Read the model definition and answer for the solid it produces. Units are mm, in the model's axes. A direction names the side the tool comes from. Coordinates: 2 decimals unless noted, no trailing zeros. Loops run counter-clockwise (first coordinate to the right, second up) from the corner with the lowest first, then second, coordinate; pieces in that order, holes last. Notation, with made-up numbers: (73.25, 12.5) - (101.25, 12.5) arc R12 ccw to (101.25, 29.5) - close; hole circle Ø10 at (3, -8). An arc over 180 degrees is marked (long way). Use one line per item in the form item = value. Start each with the question number.
1) A cutting plane is placed at D-D (x = 15.5). Give the vertices of the cut face in (y, z) (3 decimals).
2) Each of these flat-tipped pins is pushed along its axis until it touches: P1, Ø4, axis at y = 0, z = 0, coming from the +X side; P2, Ø8, axis at x = 11, y = -18, coming from the +Z side; P3, Ø8, axis at y = -10, z = -4, coming from the +X side (3 decimals); P4, Ø4, axis at x = -1, y = 0.5, coming from the -Z side. Where does it stop, or does it pass through?
3) Which of the six approach directions +Z, -Z, +X, -X, +Y, -Y give full straight-line access (tool end or side, diameter ignored) to faces 1 (the face through (-1, 0, -5.08)), 2 (the face through (14, 0, 5.08)), 3 (the face through (-6.35, -3, 2)), 4 (the face through (3.81, -3, 2))?
4) The mould has two halves that part along X. Classify faces 5 (the face through (19.05, -3, -2)), 6 (the face through (13.9, 4.1, 4.2)), 7 (the face through (6, -5.08, 0)): released by +X, released by -X, zero draft, split by the parting line, or undercut.
5) A cutting plane is placed at C-C (x = 10). Give the vertices of the cut face in (y, z) (3 decimals).
6) A cutting plane is placed at A-A (x = 6.35). Give the vertices of the cut face in (y, z) (3 decimals), and give its area (3 significant figures).
7) Consider line 1 (Y direction, x = 16, z = 0) (3 decimals); line 2 (X direction, y = -4, z = -5); line 3 (Z direction, x = 16, y = 0) (3 decimals). Determine where each line is inside the solid, lowest interval first.
Autodesk Inventor part; units mm, degrees
ref_plane "YZ Plane" through (0, 0, 0) normal (1, 0, 0) x (0, 1, 0)
ref_plane "XZ Plane" through (0, 0, 0) normal (0, 1, 0) x (-1, 0, 0)
ref_plane "XY Plane" through (0, 0, 0) normal (0, 0, 1) x (1, 0, 0)
sketch "Sketch1" plane through (0, 0, 0) normal (1, 0, 0) x (0, 1, 0)
  circle A0 centre (0, 0) radius 3.175
  line L0 (-5.08, 5.08) -> (5.08, 5.08)
  line L1 (5.08, 5.08) -> (5.08, -5.08)
  line L2 (5.08, -5.08) -> (-5.08, -5.08)
  line L3 (-5.08, -5.08) -> (-5.08, 5.08)
  line L4 (-5.08, 5.08) -> (5.08, -5.08) construction
  line L5 (5.08, 5.08) -> (-5.08, -5.08) construction
  dimension "d0" = 6.35
  dimension "d1" = 10.16
  dimension "d2" = 10.16
extrude "Extrusion1" add sketch "Sketch1" along normal blind 12.7
sketch "Sketch2" plane through (0, -5.08, -5.08) normal (0, -1, 0) x (1, 0, 0)
  line L0 (-19.05, 30.48) -> (31.75, 30.48)
  line L1 (31.75, 30.48) -> (31.75, -20.32)
  line L2 (31.75, -20.32) -> (-19.05, -20.32)
  line L3 (-19.05, -20.32) -> (-19.05, 30.48)
  line L4 (-19.05, 30.48) -> (31.75, -20.32) construction
  line L5 (31.75, 30.48) -> (-19.05, -20.32) construction
  circle A0 centre (6.35, 5.08) radius 15.875
  point P0 (0, 5.08)
  dimension "d7" = 50.8
  dimension "d8" = 50.8
  dimension "d9" = 31.75
extrude "Extrusion2" add sketch "Sketch2" along normal blind 6.35 contours A0
sketch "Sketch3" plane through (0, 5.08, 5.08) normal (0, 1, 0) x (1, 0, 0)
  line L0 (8.89, 17.78) -> (3.81, 17.78)
  line L1 (3.81, 17.78) -> (3.81, -7.62)
  line L2 (3.81, -7.62) -> (8.89, -7.62)
  line L3 (8.89, -7.62) -> (8.89, 17.78)
  line L4 (8.89, 17.78) -> (3.81, -7.62) construction
  line L5 (3.81, 17.78) -> (8.89, -7.62) construction
  line L6 (12.7, 10.16) -> (12.7, 0)
  point P0 (0, 5.08)
  point P1 (6.35, 5.08)
  dimension "d12" = 5.08
  dimension "d13" = 25.4
  dimension "d42" = 6.35
extrude "Extrusion3" cut sketch "Sketch3" against normal up to surface (10.16 mm away)
sketch "Sketch5" plane through (12.7, 0, 0) normal (1, 0, 0) x (0, 0, -1)
  line L0 (5.08, -5.08) -> (5.08, 5.08)
  line L1 (5.08, 5.08) -> (-5.08, 5.08)
  line L2 (-5.08, 5.08) -> (-5.08, -5.08)
  line L3 (-5.08, -5.08) -> (5.08, -5.08)
  circle A0 centre (0, 0) radius 3.175
extrude "Extrusion4" add sketch "Sketch5" along normal blind 6.35
sketch "Sketch6" plane through (0, 0, 0) normal (-1, 0, 0) x (0, 0, 1)
  line L0 (-5.08, -5.08) -> (-5.08, 5.08)
  line L1 (5.08, -5.08) -> (-5.08, -5.08)
  line L2 (5.08, 5.08) -> (5.08, -5.08)
  line L3 (-5.08, 5.08) -> (5.08, 5.08)
  circle A0 centre (0, 0) radius 3.175
extrude "Extrusion5" add sketch "Sketch6" along normal blind 6.35
fillet "Fillet3" radius 3.175 4 edges at (-1.27, 5.08, -5.08) (13.97, 5.08, -5.08) (-1.27, 5.08, 5.08) (13.97, 5.08, 5.08)
sketch "Sketch10" plane through (6.35, -11.43, 0) normal (0, -1, 0) x (1, 0, 0)
  circle A0 centre (0, 0) radius 15.875
  point P0 (-6.35, 0)
extrude "Extrusion9" add sketch "Sketch10" along normal blind 18.35
sketch "Sketch11" plane through (0, 0, 0) normal (1, 0, 0) x (0, 1, 0)
  line L0 (-29.78, 15.875) -> (-29.78, -15.875)
  line L1 (-29.78, 0) -> (-17.4356, 0)
  circle A0 centre (-17.4356, 0) radius 6.3
  point P0 (0, 0)
  dimension "d37" = 12.3444
  dimension "d38" = 12.6
extrude "Extrusion10" cut sketch "Sketch11" along normal mid plane 127
fillet "Fillet9" radius 3.175 4 edges at (13.97, -5.08, -5.08) (-1.27, -5.08, -5.08) (-1.27, -5.08, 5.08) (13.97, -5.08, 5.08)
properties part number "TubeMount"
Found:
q1.outline = (-29.78, -12.973) - (-5.08, -12.973) - (-5.08, -8.255) arc R3.175 cw to (-1.905, -5.08) - (1.905, -5.08) arc R3.175 ccw to (5.08, -1.905) - (5.08, 1.905) arc R3.175 ccw to (1.905, 5.08) - (-1.905, 5.08) arc R3.175 cw to (-5.08, 8.255) - (-5.08, 12.973) - (-29.78, 12.973) - close; hole circle Ø12.6 at (-17.436, 0); hole circle Ø6.35 at (0, 0)
q2.P1 = through
q2.P2 = 15.86
q2.P3 = 22.225
q2.P4 = -5.08
q3.face_1 = -Z, +X, -X, +Y
q3.face_2 = +Z, +X, -X, +Y
q3.face_3 = +Z, -Z, -X, +Y
q3.face_4 = +Z, -Z, +Y
q4.face_5 = released by +X
q4.face_6 = zero draft
q4.face_7 = undercut
q5.outline = (-29.78, -15.45) - (-5.08, -15.45) - (-5.08, -8.255) arc R3.175 cw to (-1.905, -5.08) - (1.905, -5.08) arc R3.175 ccw to (5.08, -1.905) - (5.08, 1.905) arc R3.175 ccw to (1.905, 5.08) - (-1.905, 5.08) arc R3.175 cw to (-5.08, 8.255) - (-5.08, 15.45) - (-29.78, 15.45) - close; hole circle Ø12.6 at (-17.436, 0); hole circle Ø6.35 at (0, 0)
q6.outline = (-29.78, -15.875) - (-5.08, -15.875) - (-5.08, 15.875) - (-29.78, 15.875) - close; hole circle Ø12.6 at (-17.436, 0)
q6.area = 660 mm^2
q7.line_1 = -29.78 to -23.736, -11.136 to -3.175, 3.175 to 5.08
q7.line_2 = -6.35 to 3.81, 8.89 to 19.05
q7.line_3 = -5.08 to -3.175, 3.175 to 5.08
